Study the drawing (mm; zero at the part's minimum x, y, z) and answer. A direction names the side the tool comes from. Round coordinates to 2 decimals unless told otherwise and drop trailing zeros. Loops run counter-clockwise (first coordinate to the right, second up) from the corner with the lowest first, then second, coordinate; pieces in that order, holes last. Notation, with made-up numbers: M -9.75,39 L 35.25,39 A24 cw 35.25,70 Z; hole C 38.5,4 d1. An arc over 180 degrees is marked long. Put each result on its own line as item: value. Start each with the question number.
(1) Straight lines are drawn through the part: line 1 (Z direction, x = 60, y = 91.5); line 2 (Z direction, x = 60.5, y = 89); line 3 (Y direction, x = 81.5, z = 10.75). For each, find the intervals that lie inside material, in ascending order.
(2) Flat-ended cylindrical pins translate along their axes: P1, Ø2, axis at y = 31, z = 10.5, coming from the -X side; P2, Ø4, axis at x = 19, z = 7.5, coming from the -Y side; P3, Ø25, axis at x = 18, y = 86.5, coming from the +Z side. Find the tip coordinate at first contact, or state that the pin passes through.
(3) Section A-A, the plane x = 11.5 is taken. Determine the outline of the cut face in (y, z), then the cut area to 3 significant figures.
(4) Section D-D, the plane x = 45.5 is taken. Determine the outline of the cut face in (y, z).
(5) Section B-B, the plane z = 17.25 is taken. Determine the outline of the cut face in (x, y) (1 decimal).
(6) Section C-C, the plane y = 76.5 is taken. Determine the outline of the cut face in (x, z), then the cut area to 3 significant figures.
(7) Which of the six approach directions +Z, -Z, +X, -X, +Y, -Y give full straight-line access (tool end or side, diameter ignored) to the marked faces 1, 2, 3 and 4?
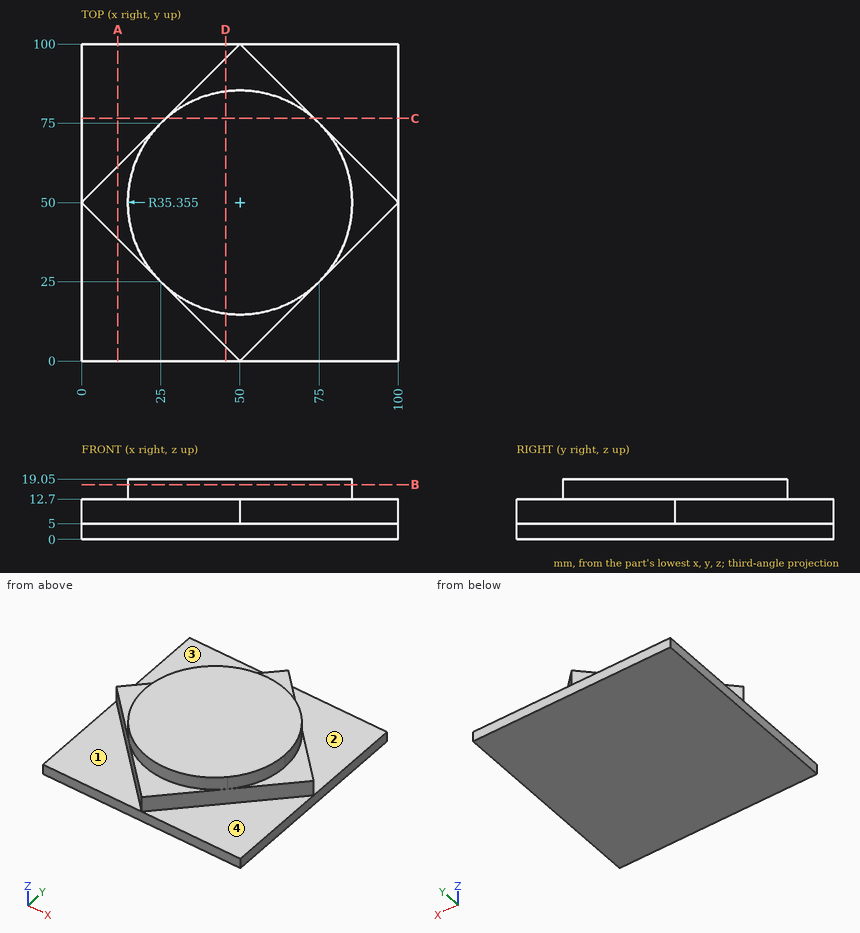
Recorded:
1. line 1: z = 0 to 5
1. line 2: z = 0 to 12.7
1. line 3: y = 31.5 to 68.5
2. P1: stops at x = 18
2. P2: stops at y = 29
2. P3: stops at z = 5
3. outline: M 0,0 L 100,0 L 100,5 L 61.5,5 L 61.5,12.7 L 38.5,12.7 L 38.5,5 L 0,5 Z
3. area: 677 mm²
4. outline: M 0,0 L 100,0 L 100,5 L 95.5,5 L 95.5,12.7 L 85.07,12.7 L 85.07,19.05 L 14.93,19.05 L 14.93,12.7 L 4.5,12.7 L 4.5,5 L 0,5 Z
5. outline: C 50,50 d70.7
6. outline: M 0,0 L 100,0 L 100,5 L 73.5,5 L 73.5,12.7 L 73.4,12.7 L 73.4,19.05 L 26.6,19.05 L 26.6,12.7 L 26.5,12.7 L 26.5,5 L 0,5 Z
6. area: 1,160 mm²
7. face 1: +Z, -X, -Y
7. face 2: +Z, +X, +Y
7. face 3: +Z, -X, +Y
7. face 4: +Z, +X, -Y
